Geometry check sheet. Reference: the model listing, model coordinates, mm. A direction names the side the tool comes from. Give positions to 0.01 mm unless a question says otherwise; leave off trailing zeros. Write each loop counter-clockwise with the first axis right and the second up, starting at its lowest first coordinate (ties: lowest second). Pieces come first, ordered by that corner, then holes. Notation, with made-up numbers: M 0.25,-9 L 47.25,-9 A29 cw 47.25,15 Z; hole C 40.5,-15 d8. An arc over 180 degrees is marked long. One line per item, written item: value. Start each with the question number.
1. Scan lines: line 1 (Y direction, x = -2, z = -5); line 2 (X direction, y = 3.5, z = -5.5); line 3 (Z direction, x = -2.25, y = 7). Record each from-to range of solid material in increasing order.
2. Cross-section at B-B on z = -15. Record the cut outline in (x, y).
3. Tool access check on faces 1 (the face through (-5.9, 5, -3.7)), 2 (the face through (0, 4, -8)), 3 (the face through (-4, 2, -10)). Record the directions out of +Z, -Z, +X, -X, +Y, -Y that give a thin tool (end or side, any length) a straight path to the whole face; none if there is none.
4. Cross-section at A-A on x = -3. Record the cut outline in (y, z).
5. Gauge pin test, flat ends, axial feed: pin 1 (4 mm diameter, centred on x = -8, y = 7.5, fed in from -Z); pin 2 (1.2 mm diameter, centred on y = 6.5, z = -10.5, fed in from -X). Record the tip position at first contact, or that the pin passes through.
Autodesk Inventor part; units mm, degrees
ref_plane "YZ Plane" through (0, 0, 0) normal (1, 0, 0) x (0, 1, 0)
ref_plane "XZ Plane" through (0, 0, 0) normal (0, 1, 0) x (-1, 0, 0)
ref_plane "XY Plane" through (0, 0, 0) normal (0, 0, 1) x (1, 0, 0)
sketch "Sketch1" plane through (0, 0, 0) normal (0, 1, 0) x (-1, 0, 0)
  line L0 (0, 0) -> (16.7, 0)
  line L1 (16.7, 0) -> (16.7, -4)
  line L2 (16.7, -4) -> (4, -4)
  line L3 (4, -4) -> (4, -16.7)
  line L4 (4, -16.7) -> (0, -16.7)
  line L5 (0, -16.7) -> (0, 0)
  dimension "d0" = 16.7
  dimension "d1" = 4
  dimension "d2" = 4
  dimension "d3" = 16.7
extrude "Extrusion1" add sketch "Sketch1" along normal blind 5
sketch "Sketch2" plane through (0, 5, 0) normal (0, 1, 0) x (1, 0, 0)
  line L0 (-16.7, 4) -> (-16.7, 0)
  line L1 (-16.7, 0) -> (-16.7, 1.8)
  line L2 (-16.7, 1.8) -> (-1.8, 1.8)
  line L3 (-1.8, 1.8) -> (-1.8, 16.7)
  line L4 (-1.8, 16.7) -> (0, 16.7)
  line L5 (-16.7, 0) -> (0, 0)
  line L6 (0, 16.7) -> (0, 0)
  line L7 (-16.7, 0) -> (0, 0)
  dimension "d6" = 1.8
  dimension "d7" = 1.8
  dimension "d8" = 16.7
extrude "Extrusion2" add sketch "Sketch2" along normal blind 4
properties part number "TestingPlatform_stackFeet01"
Report:
1. line 1: y = 0 to 5
1. line 2: x = -4 to 0
1. line 3: z = -1.8 to 0
2. outline: M -4,0 L 0,0 L 0,9 L -1.8,9 L -1.8,5 L -4,5 Z
3. face 1: -Z, -X, +Y
3. face 2: +Z, -Z, +X, +Y, -Y
3. face 3: -Z, -X, +Y, -Y
4. outline: M 0,-16.7 L 5,-16.7 L 5,-1.8 L 9,-1.8 L 9,0 L 0,0 Z
5. pin 1: stops at z = -1.8
5. pin 2: stops at x = -1.8
